```python
from build123d import *

# Parameters (mm, degrees)
SKETCH1_R           = 50.8
SKETCH1_R_2         = 6.5024
SKETCH1_R_3         = 12.7
BOSS_EXTRUDE1_DEPTH = 9.525
SKETCH2_R           = 49.276
SKETCH2_R_2         = 44.45
BOSS_EXTRUDE2_DEPTH = 63.5
SKETCH3_R           = 12.7
SKETCH3_R_2         = 6.5024
BOSS_EXTRUDE3_DEPTH = 15.875
CHAMFER1_SIZE       = 6.35
CHAMFER1_SIZE2      = 2.54
SKETCH4_R           = 12.7
SKETCH4_R_2         = 6.5024
BOSS_EXTRUDE4_DEPTH = 6.35
FILLET1_R           = 2.54


with BuildPart() as part:
    # Sketch1 → Boss-Extrude1 (new body)
    with BuildSketch(Plane(origin=(0, 0, 0), x_dir=(1, 0, 0), z_dir=(0, 1, 0))):
        Circle(SKETCH1_R)
        Circle(SKETCH1_R_2, mode=Mode.SUBTRACT)
        with Locations((0, 28.575)):
            Circle(SKETCH1_R_3, mode=Mode.SUBTRACT)
        with Locations((27.176439953, 8.830160614)):
            Circle(SKETCH1_R_3, mode=Mode.SUBTRACT)
        with Locations((16.795963584, -23.117660614)):
            Circle(SKETCH1_R_3, mode=Mode.SUBTRACT)
        with Locations((-16.795963584, -23.117660614)):
            Circle(SKETCH1_R_3, mode=Mode.SUBTRACT)
        with Locations((-27.176439953, 8.830160614)):
            Circle(SKETCH1_R_3, mode=Mode.SUBTRACT)
    extrude(amount=BOSS_EXTRUDE1_DEPTH)

    # Sketch2 → Boss-Extrude2 (add)
    with BuildSketch(Plane(origin=(0, 9.525, 0), x_dir=(1, 0, 0), z_dir=(0, 1, 0))):
        Circle(SKETCH2_R)
        Circle(SKETCH2_R_2, mode=Mode.SUBTRACT)
    extrude(amount=BOSS_EXTRUDE2_DEPTH)

    # Sketch3 → Boss-Extrude3 (add)
    with BuildSketch(Plane(origin=(0, 9.525, 0), x_dir=(1, 0, 0), z_dir=(0, 1, 0))):
        Circle(SKETCH3_R)
        Circle(SKETCH3_R_2, mode=Mode.SUBTRACT)
    extrude(amount=BOSS_EXTRUDE3_DEPTH)

    # Chamfer1
    chamfer1_edges = [part.edges().sort_by_distance(p)[0] for p in [
        (-49.276, 73.025, 0),
    ]]
    chamfer1_side = [part.faces().sort_by_distance(p)[0] for p in [
        (-49.276, 41.275, 0),
    ]]
    chamfer(chamfer1_edges, length=CHAMFER1_SIZE, length2=CHAMFER1_SIZE2, reference=chamfer1_side[0])

    # Sketch4 → Boss-Extrude4 (add)
    with BuildSketch(Plane(origin=(0, 25.4, 0), x_dir=(1, 0, 0), z_dir=(0, 1, 0))):
        Circle(SKETCH4_R)
        Circle(SKETCH4_R_2, mode=Mode.SUBTRACT)
    extrude(amount=BOSS_EXTRUDE4_DEPTH)

    # Fillet1
    fillet1_edges = [part.edges().sort_by_distance(p)[0] for p in [
        (-12.7, 31.75, 0),
    ]]
    fillet(fillet1_edges, radius=FILLET1_R)


solid = part.part
```
Geometry check sheet. Reference: the model listing, model coordinates, mm. A direction names the side the tool comes from. Give positions to 0.01 mm unless a question says otherwise; leave off trailing zeros. Write each loop counter-clockwise with the first axis right and the second up, starting at its lowest first coordinate (ties: lowest second). Pieces come first, ordered by that corner, then holes. Notation, with made-up numbers: (-12.75, -11.75) -> (31.25, -11.75) arc R22 cw to (31.25, 16.25) -> close; hole circle Ø5 at (80.25, 2.5). An arc over 180 degrees is marked (long way). Use one line per item in the form item = value.
Item 1: Sectioned sample at B-B on z = 0. Count the separate pieces of the cut face and the enclosed holes in it, plus the area to 3 significant figures.
Results list:
separate_pieces = 4
enclosed_holes = 0
area = 1,370 mm2
Item 2: Mould release check, pull along X, two halves, no side actions. Record for faces 3 (the cylindrical face through (-0.846, 15.653, -6.447)), 4 (the conical face through (21.62, 72.72, 41.57)), 5 (the flat face through (-42, 9.525, -27)): released by +X, released by -X, zero draft, split by the parting line, or undercut.
Results list:
face_3 = undercut
face_4 = split by the parting line
face_5 = zero draft
Item 3: Access from +Z, -Z, +X, -X, +Y, -Y to the whole of each face (thin tool, end or side, straight path). Record for faces 1 (the cylindrical face through (-11.012, 4.696, 49.592)), 2 (the cylindrical face through (42.397, 40.83, -13.352)).
Results list:
face_1 = +Y, -Y
face_2 = +Y
Item 4: Scan lines: line 1 (X direction, y = 34, z = 0); line 2 (Z direction, x = 7.5, y = 3.5). Record each from-to range of solid material in increasing order.
Results list:
line_1 = -49.28 to -44.45, 44.45 to 49.28
line_2 = -50.24 to -38.82, -18.33 to 14.46, 31.77 to 50.24
Item 5: Depth check by flat-ended pin: pin 1 Ø22.5 at (x, z) = (2.5, 1.5) entering from +Y; pin 2 Ø8 at (y, z) = (61, 24) entering from +X; pin 3 Ø6 at (x, y) = (12.5, 58) entering from -Z; pin 4 Ø17 at (x, z) = (0, 0) entering from -Y. Enter the tip coordinate at first touch or a pass-through.
Results list:
pin_1 = 31.75
pin_2 = 45.03
pin_3 = -48.35
pin_4 = 0
Item 6: Sectioned sample at C-C on y = 11.5. Enter the section's corners in (x, z).
Results list:
outline = circle Ø98.55 at (0, 0); circle Ø25.4 at (0, 0); hole circle Ø88.9 at (0, 0); hole circle Ø13 at (0, 0)
Item 7: Sectioned sample at A-A on x = 0. Enter the section's corners in (y, z) (3 decimals).
Results list:
outline = (0, -50.8) -> (9.525, -50.8) -> (9.525, -49.276) -> (66.675, -49.276) -> (73.025, -46.736) -> (73.025, -44.45) -> (9.525, -44.45) -> (9.525, -41.275) -> (0, -41.275) -> close; (0, -15.875) -> (9.525, -15.875) -> (9.525, -12.7) -> (29.21, -12.7) arc R2.54 ccw to (31.75, -10.16) -> (31.75, -6.502) -> (0, -6.502) -> close; (0, 6.502) -> (31.75, 6.502) -> (31.75, 10.16) arc R2.54 ccw to (29.21, 12.7) -> (9.525, 12.7) -> (9.525, 44.45) -> (73.025, 44.45) -> (73.025, 46.736) -> (66.675, 49.276) -> (9.525, 49.276) -> (9.525, 50.8) -> (0, 50.8) -> close
Item 8: Sectioned sample at D-D on y = 57. Enter the section's corners in (x, z).
Results list:
outline = circle Ø98.55 at (0, 0); hole circle Ø88.9 at (0, 0)
